Geometry check sheet. Reference: drawing and pictorial views, mm from the part's lowest x, y, z. Give positions to 0.01 mm unless a question says otherwise; leave off trailing zeros. Order: outer loops, then holes, each group sorted by start corner. A loop starts at its lowest first (then second) coordinate and runs counter-clockwise, first axis right, second up. Notation, with made-up numbers: (66.5, 66.25) -> (119.5, 66.25) arc R19 ccw to (119.5, 101.25) -> close; hole circle Ø1 at (16, -23). An arc over 180 degrees is marked (long way). Write each question's results on one line, items separated by ' | '.
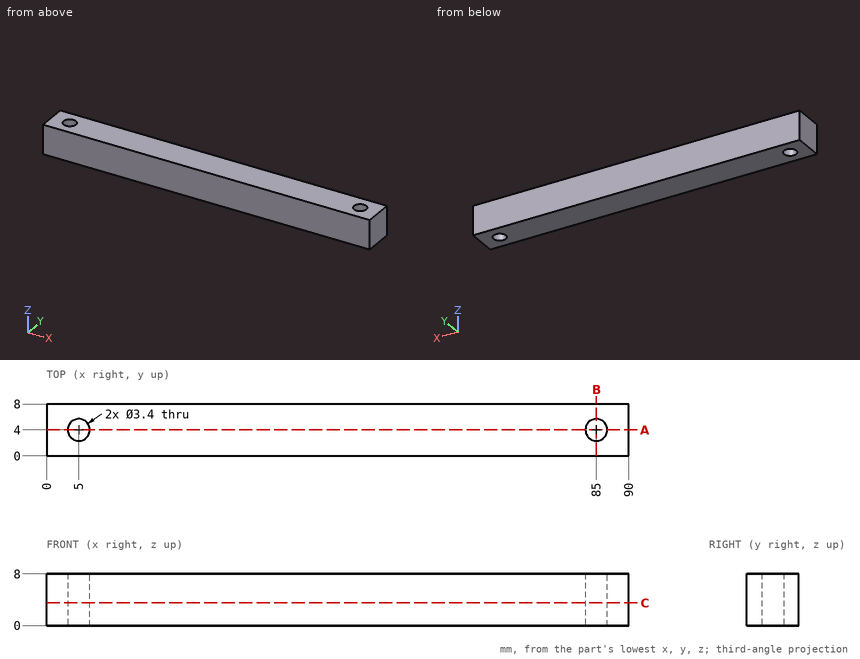
1. Section check C-C on z = 3.5. Record the cut outline in (x, y).
Verdict:
outline: (0, 0) -> (90, 0) -> (90, 8) -> (0, 8) -> close; hole circle Ø3.4 at (5, 4); hole circle Ø3.4 at (85, 4)
2. Section check A-A on y = 4. Record the cut outline in (x, z).
Verdict:
outline: (0, 0) -> (3.3, 0) -> (3.3, 8) -> (0, 8) -> close; (6.7, 0) -> (83.3, 0) -> (83.3, 8) -> (6.7, 8) -> close; (86.7, 0) -> (90, 0) -> (90, 8) -> (86.7, 8) -> close
3. Section check B-B on x = 85. Record the cut outline in (y, z).
Verdict:
outline: (0, 0) -> (2.3, 0) -> (2.3, 8) -> (0, 8) -> close; (5.7, 0) -> (8, 0) -> (8, 8) -> (5.7, 8) -> close
4. Material ranges on probe 1 along X at (y, z) = (4.25, 5.75); probe 2 along Y at (x, z) = (85, 5.75); probe 3 along X at (y, z) = (4.75, 6.5), recorded low to high. Write a range as from..to.
Verdict:
probe 1: x = 0..3.32, 6.68..83.32, 86.68..90 | probe 2: y = 0..2.3, 5.7..8 | probe 3: x = 0..3.47, 6.53..83.47, 86.53..90
